Model file for the job. Use its own axes, mm. A direction names the side the tool comes from. Coordinates: 2 decimals unless noted, no trailing zeros. Loops run counter-clockwise (first coordinate to the right, second up) from the corner with the lowest first, then second, coordinate; pieces in that order, holes last. Notation, with made-up numbers: (-18.75, -24.75) -> (31.25, -24.75) arc R27 ccw to (31.25, -3.75) -> close; hole circle Ø2 at (61, 80). An arc over 180 degrees is marked (long way). Use one line per item in the form item = value.
```python
from build123d import *

# Parameters (mm, degrees)
SKETCH_1_R               = 27.5
EXTRUDE_1_DEPTH          = 10
SKETCH_2_R               = 2.75
CUT_EXTRUDE_1_DEPTH      = 10
PATTERN_CIRCULAR_1_COUNT = 2
SKETCH_3_R               = 6
EXTRUDE_2_DEPTH          = 22
SKETCH_5_R               = 3.15
CUT_EXTRUDE_3_DEPTH      = 12
SKETCH_4_R               = 4.05
CUT_EXTRUDE_2_DEPTH      = 15
CUT_EXTRUDE_4_DEPTH      = 45.682211225
CUT_EXTRUDE_4_DEPTH_BACK = 45.682211225
SKETCH_6_R               = 2


with BuildPart() as part:
    # 草图1 → 凸台-拉伸1 (new body)
    with BuildSketch(Plane(origin=(0, 0, 0), x_dir=(1, 0, 0), z_dir=(0, 1, 0))):
        with Locations(Location((0, 0, 0), (0, 0, 270))):
            Circle(SKETCH_1_R)
    extrude(amount=EXTRUDE_1_DEPTH)

    # 草图2 → 切除-拉伸1 (cut)
    with BuildSketch(Plane.XZ):
        with Locations(Location((18.515, 0, 0), (0, 0, 270))):
            Circle(SKETCH_2_R)
    cut_extrude_1 = extrude(amount=-CUT_EXTRUDE_1_DEPTH, mode=Mode.SUBTRACT)

    # 阵列(圆周)1: 切除-拉伸1 ×2 about axis
    pattern_circular_1_axis = Axis((0, 0, 0), (0, 1, 0))
    for i in range(1, PATTERN_CIRCULAR_1_COUNT):
        add(cut_extrude_1.rotate(pattern_circular_1_axis, i * 360 / PATTERN_CIRCULAR_1_COUNT), mode=Mode.SUBTRACT)

    # 草图3 → 凸台-拉伸2 (add)
    with BuildSketch(Plane.XZ):
        with Locations(Location((0, 0, 0), (0, 0, 270))):
            Circle(SKETCH_3_R)
    extrude(amount=EXTRUDE_2_DEPTH)

    # 草图5 → 切除-拉伸3 (cut)
    with BuildSketch(Plane.XZ.offset(22)):
        with Locations(Location((0, 0, 0), (0, 0, 270))):
            Circle(SKETCH_5_R)
    extrude(amount=-CUT_EXTRUDE_3_DEPTH, mode=Mode.SUBTRACT)

    # 草图4 → 切除-拉伸2 (cut)
    with BuildSketch(Plane(origin=(0, 10, 0), x_dir=(1, 0, 0), z_dir=(0, 1, 0))):
        with Locations(Location((0, 0, 0), (0, 0, 270))):
            Circle(SKETCH_4_R)
    extrude(amount=-CUT_EXTRUDE_2_DEPTH, mode=Mode.SUBTRACT)

    # 草图6 → 切除-拉伸4 (cut, two sides: drawn at the far end of the back side and taken through both)
    with BuildSketch(Plane.XY.offset(-CUT_EXTRUDE_4_DEPTH_BACK)):
        with Locations((0, -18)):
            Circle(SKETCH_6_R)
    extrude(amount=CUT_EXTRUDE_4_DEPTH + CUT_EXTRUDE_4_DEPTH_BACK, mode=Mode.SUBTRACT)


solid = part.part
```
Q1. Band-saw the part on C-C, the plane y = -18. Write the cut outline in (x, z).
Result:
outline = (-2, -5.66) -> (-2, -2.43) arc R3.15 cw to (-2, 2.43) -> (-2, 5.66) arc R6 ccw to start; (2, -5.66) arc R6 ccw to (2, 5.66) -> (2, 2.43) arc R3.15 cw to (2, -2.43) -> close
Q2. Band-saw the part on B-B, the plane z = 0. Write the cut outline in (x, y) (3 decimals).
Result:
outline = (-27.5, 0) -> (-21.265, 0) -> (-21.265, 10) -> (-27.5, 10) -> close; (-15.765, 0) -> (-6, 0) -> (-6, -22) -> (-3.15, -22) -> (-3.15, -10) -> (3.15, -10) -> (3.15, -22) -> (6, -22) -> (6, 0) -> (15.765, 0) -> (15.765, 10) -> (4.05, 10) -> (4.05, -5) -> (-4.05, -5) -> (-4.05, 10) -> (-15.765, 10) -> close; (21.265, 0) -> (27.5, 0) -> (27.5, 10) -> (21.265, 10) -> close
Q3. Pin check, flat tips, straight feed: pin 1 Ø4 at (y, z) = (5.5, -10.5) entering from +X; pin 2 Ø1.5 at (y, z) = (0, -21.5) entering from +X; pin 3 Ø5 at (x, y) = (0, -18) entering from -Z; pin 4 Ø5 at (x, z) = (18.515, 0) entering from +Y. Stop position of each tip, or through.
Result:
pin_1 = 26.15
pin_2 = 18.05
pin_3 = -6
pin_4 = through
Q4. Wall check: line 1 along X through (y, z) = (5.75, 0) (3 decimals); line 2 along X through (y, z) = (-14, 0); line 3 along Y through (x, z) = (-17.5, 13.5). Give the ranges that are in metal, low to high.
Result:
line_1 = -27.5 to -21.265, -15.765 to -4.05, 4.05 to 15.765, 21.265 to 27.5
line_2 = -6 to -3.15, 3.15 to 6
line_3 = 0 to 10
Q5. Band-saw the part on A-A, the plane x = 0. Write the cut outline in (y, z).
Result:
outline = (-22, -6) -> (-20, -6) -> (-20, -3.15) -> (-22, -3.15) -> close; (-22, 3.15) -> (-20, 3.15) -> (-20, 6) -> (-22, 6) -> close; (-16, -6) -> (0, -6) -> (0, -27.5) -> (10, -27.5) -> (10, -4.05) -> (-5, -4.05) -> (-5, 4.05) -> (10, 4.05) -> (10, 27.5) -> (0, 27.5) -> (0, 6) -> (-16, 6) -> (-16, 3.15) -> (-10, 3.15) -> (-10, -3.15) -> (-16, -3.15) -> close
Q6. Mould opens along Z. For faces 1 (the face through (-21.24, 4.93, -0.36)), 2 (the face through (-5.323, -10.846, -2.769)), 3 (the face through (0, -16, 4)) say: released by +Z, released by -Z, zero draft, split by the parting line, or undercut.
Result:
face_1 = undercut
face_2 = split by the parting line
face_3 = zero draft
Q7. Band-saw the part on D-D, the plane y = -4. Write the cut outline in (x, z), and give its area (3 significant figures).
Result:
outline = circle Ø12 at (0, 0); hole circle Ø8.1 at (0, 0)
area = 61.6 mm2
Q8. Which spindle directions (+Z, -Z, +X, -X, +Y, -Y) get a long thin tool onto all of the face, cutting with end or side? Do faces 4 (the face through (-24.397, 4.93, 12.69)), 5 (the face through (0, -5, 0)), 6 (the face through (0, -10, 0)). Say none if no direction does.
Result:
face_4 = +Y, -Y
face_5 = +Y
face_6 = -Y
